Here's how the part is built. I have some questions about the finished solid (model axes, mm). A direction names the side the tool comes from. Round coordinates to 2 decimals unless told otherwise and drop trailing zeros. Loops run counter-clockwise (first coordinate to the right, second up) from the corner with the lowest first, then second, coordinate; pieces in that order, holes last. Notation, with made-up numbers: M 12.5,26 L 42.5,26 A23 ccw 42.5,62 Z; hole C 38.25,55.5 d3. An arc over 180 degrees is marked long. Answer as CSV lines item,"result".
```python
from build123d import *

# Parameters (mm, degrees)
F2_W      = 40
F2_H      = 40
F7_W      = 32
F7_H      = 32
F13_DEPTH = 1
F14_START = -2
F14_DEPTH = 3
F16_DEPTH = 1
F17_START = -2
F17_DEPTH = 3
F19_DEPTH = 1
F20_START = -2
F20_DEPTH = 3
F22_DEPTH = 1
F23_START = -2
F23_DEPTH = 3


with BuildPart() as f5:
    # F2 (on Top) → F5 section 0
    with BuildSketch(Plane.XY, mode=Mode.PRIVATE) as f5_s0:
        Rectangle(F2_W, F2_H)
    loft([f5_s0.sketch, Vertex(0, 0, 28.2842712475)])

    # F7 (on Top) → F9 section 0
    with BuildSketch(Plane.XY, mode=Mode.PRIVATE) as f9_s0:
        Rectangle(F7_W, F7_H)
    loft([f9_s0.sketch, Vertex(0, 0, 22.627416998)], mode=Mode.SUBTRACT)

    # F12 (on offset) → F13 (cut)
    with BuildSketch(Plane(origin=(0, -13.3333333333, 9.4280904158), x_dir=(1, 0, 0), z_dir=(0, -0.8164965809, 0.5773502692))):
        Polygon((13.0717967697, -5.5470053838), (0, 17.0940107676), (-13.0717967697, -5.5470053838), align=None)
    extrude(amount=-F13_DEPTH, mode=Mode.SUBTRACT)

    # F12 (on offset) → F14 (cut)
    with BuildSketch(Plane(origin=(0, -13.3333333333, 9.4280904158), x_dir=(1, 0, 0), z_dir=(0, -0.8164965809, 0.5773502692)).offset(F14_START)):
        Polygon((13.0717967697, -5.5470053838), (0, 17.0940107676), (-13.0717967697, -5.5470053838), align=None)
    extrude(amount=-F14_DEPTH, mode=Mode.SUBTRACT)

    # F15 (on offset) → F16 (cut)
    with BuildSketch(Plane(origin=(-13.3333333333, 0, 9.4280904158), x_dir=(0, -1, 0), z_dir=(-0.8164965809, 0, 0.5773502692))):
        Polygon((13.0717967697, -5.5470053838), (0, 17.0940107676), (-13.0717967697, -5.5470053838), align=None)
    extrude(amount=-F16_DEPTH, mode=Mode.SUBTRACT)

    # F15 (on offset) → F17 (cut)
    with BuildSketch(Plane(origin=(-13.3333333333, 0, 9.4280904158), x_dir=(0, -1, 0), z_dir=(-0.8164965809, 0, 0.5773502692)).offset(F17_START)):
        Polygon((13.0717967697, -5.5470053838), (0, 17.0940107676), (-13.0717967697, -5.5470053838), align=None)
    extrude(amount=-F17_DEPTH, mode=Mode.SUBTRACT)

    # F18 (on face) → F19 (cut)
    with BuildSketch(Plane(origin=(0, 13.3333333333, 9.4280904158), x_dir=(-1, 0, 0), z_dir=(0, 0.8164965809, 0.5773502692))):
        Polygon((13.0717967697, -5.5470053838), (0, 17.0940107676), (-13.0717967697, -5.5470053838), align=None)
    extrude(amount=-F19_DEPTH, mode=Mode.SUBTRACT)

    # F18 (on face) → F20 (cut)
    with BuildSketch(Plane(origin=(0, 13.3333333333, 9.4280904158), x_dir=(-1, 0, 0), z_dir=(0, 0.8164965809, 0.5773502692)).offset(F20_START)):
        Polygon((13.0717967697, -5.5470053838), (0, 17.0940107676), (-13.0717967697, -5.5470053838), align=None)
    extrude(amount=-F20_DEPTH, mode=Mode.SUBTRACT)

    # F21 (on face) → F22 (cut)
    with BuildSketch(Plane(origin=(13.3333333333, 0, 9.4280904158), x_dir=(0, 1, 0), z_dir=(0.8164965809, 0, 0.5773502692))):
        Polygon((13.0717967697, -5.5470053838), (0, 17.0940107676), (-13.0717967697, -5.5470053838), align=None)
    extrude(amount=-F22_DEPTH, mode=Mode.SUBTRACT)

    # F21 (on face) → F23 (cut)
    with BuildSketch(Plane(origin=(13.3333333333, 0, 9.4280904158), x_dir=(0, 1, 0), z_dir=(0.8164965809, 0, 0.5773502692)).offset(F23_START)):
        Polygon((13.0717967697, -5.5470053838), (0, 17.0940107676), (-13.0717967697, -5.5470053838), align=None)
    extrude(amount=-F23_DEPTH, mode=Mode.SUBTRACT)


solid = f5.part
```
1. If I drill on line 1 (X direction, y = 2.5, z = 3); line 2 (Y direction, x = -1.5, z = 9); line 3 (Y direction, x = -8, z = 9.75), over which ranges is the centre line in solid material (lowest first)? Write a range as [from, to].
Evaluation:
line 1,"x = [-17.88, -13.88], [13.88, 17.88]"
line 2,"y = [-12.41, -11.19], [11.19, 12.41]"
line 3,"y = [-11.88, -10.66], [10.66, 11.88]"
2. I want a section at A-A, the plane z = 2.25. Please give me the cut outline in (x, y), and give its area (3 significant figures).
Evaluation:
outline,"M -18.41,-18.41 L 18.41,-18.41 L 18.41,18.41 L -18.41,18.41 Z; hole M -14.41,-14.41 L 14.41,-14.41 L 14.41,14.41 L -14.41,14.41 Z"
area,"525 mm²"
3. Which directions (+Z, -Z, +X, -X, +Y, -Y) give clear straight access to the entire face, cutting with the end or side of a thin tool? Please do faces 4 (the flat face through (9.7, -0.2, 11.1)), 5 (the flat face through (-0.093, -17.361, 3.732)).
Evaluation:
face 4,"none"
face 5,"+Z, +X, -X, -Y"
4. We'd pull the mould along Z, two halves only. Please class faces 1 (the flat face through (0.18, 14.39, 3.38)), 2 (the flat face through (-14.48, 1.26, 2.15)), 3 (the flat face through (17.361, -0.093, 3.732)): pulls with the +Z half, pulls with the -Z half, needs draft (parallel to the pull), parting line crosses it, or undercut.
Evaluation:
face 1,"undercut"
face 2,"pulls with the -Z half"
face 3,"pulls with the +Z half"
5. For P1, Ø5, axis at x = 8.5, y = -0.5, coming from the -Z side; P2, Ø6, axis at x = 14.5, y = -7, coming from the -Z side; P3, Ø8, axis at x = 3.5, y = 8, coming from the +Z side; P4, Ø12, axis at y = 12, z = 14.5, coming from the -X side, each with a flat end and sliding along its axis, tell me the tip position at first contact or that it passes through.
Evaluation:
P1,"stops at z = 9.26"
P2,"stops at z = 0"
P3,"stops at z = 22.63"
P4,"stops at x = -13.99"
6. I want a section at D-D, the plane z = 24. Please give me the cut outline in (x, y), and give its area (3 significant figures).
Evaluation:
outline,"M -3.03,-3.03 L 3.03,-3.03 L 3.03,3.03 L -3.03,3.03 Z"
area,"36.7 mm²"
